Check sheet for the modelled part. Datum: model origin and axes. Units: mm. Coordinates: 2 decimals unless noted, no trailing zeros. Loops run counter-clockwise (first coordinate to the right, second up) from the corner with the lowest first, then second, coordinate; pieces in that order, holes last. Notation, with made-up numbers: (-8.75, 71.25) -> (36.25, 71.25) arc R11 ccw to (36.25, 86.25) -> close; hole circle Ø1 at (52, 67). An arc over 180 degrees is marked (long way). Use one line per item in the form item = value.
from build123d import *

# Parameters (mm, degrees)
F0_W     = 112
F0_H     = 94
F0_W_2   = 3
F0_H_2   = 10
F0_W_3   = 10
F0_H_3   = 3
F0_R     = 1.5
F1_DEPTH = 3


with BuildPart() as f1:
    # F0 (on Front) → F1 (new body)
    with BuildSketch(Plane.XZ):
        Rectangle(F0_W, F0_H)
        with Locations((-51.5, -7)):
            Rectangle(F0_W_2, F0_H_2, mode=Mode.SUBTRACT)
        with Locations((0, -42.5)):
            Rectangle(F0_W_3, F0_H_3, mode=Mode.SUBTRACT)
        with Locations((51.5, -7)):
            Rectangle(F0_W_2, F0_H_2, mode=Mode.SUBTRACT)
        with Locations((-51.5, 3)):
            Circle(F0_R, mode=Mode.SUBTRACT)
        with Locations((-51.5, 13)):
            Rectangle(F0_W_2, F0_H_2, mode=Mode.SUBTRACT)
        with Locations((51.5, 3)):
            Circle(F0_R, mode=Mode.SUBTRACT)
        with Locations((51.5, 13)):
            Rectangle(F0_W_2, F0_H_2, mode=Mode.SUBTRACT)
    extrude(amount=F1_DEPTH)


solid = f1.part
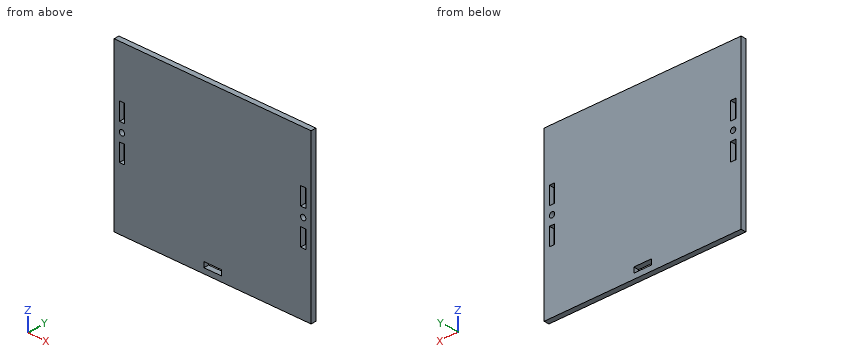
(1) Section check B-B, the plane z = 3. Record the boundary of the cut face in (x, y), plus the area to 3 significant figures.
Established:
outline = (-56, -3) -> (-53, -3) -> (-53, 0) -> (-56, 0) -> close; (-50, -3) -> (50, -3) -> (50, 0) -> (-50, 0) -> close; (53, -3) -> (56, -3) -> (56, 0) -> (53, 0) -> close
area = 318 mm²
(2) Section check D-D, the plane x = -1. Record the boundary of the cut face in (y, z).
Established:
outline = (-3, -47) -> (0, -47) -> (0, -44) -> (-3, -44) -> close; (-3, -41) -> (0, -41) -> (0, 47) -> (-3, 47) -> close
(3) Scan lines: line 1 along Z through (x, y) = (51.5, -2.15); line 2 along X through (y, z) = (-2.45, -7); line 3 along Z through (x, y) = (4, -2.85). Record each from-to range of solid material in increasing order.
Established:
line_1 = -47 to -12, -2 to 1.5, 4.5 to 8, 18 to 47
line_2 = -56 to -53, -50 to 50, 53 to 56
line_3 = -47 to -44, -41 to 47
(4) Section check A-A, the plane x = -51.5. Record the boundary of the cut face in (y, z), plus the area to 3 significant figures.
Established:
outline = (-3, -47) -> (0, -47) -> (0, -12) -> (-3, -12) -> close; (-3, -2) -> (0, -2) -> (0, 1.5) -> (-3, 1.5) -> close; (-3, 4.5) -> (0, 4.5) -> (0, 8) -> (-3, 8) -> close; (-3, 18) -> (0, 18) -> (0, 47) -> (-3, 47) -> close
area = 213 mm²
(5) Section check C-C, the plane y = -1.65. Record the boundary of the cut face in (x, z).
Established:
outline = (-56, -47) -> (56, -47) -> (56, 47) -> (-56, 47) -> close; hole (-53, -12) -> (-50, -12) -> (-50, -2) -> (-53, -2) -> close; hole circle Ø3 at (-51.5, 3); hole (-53, 8) -> (-50, 8) -> (-50, 18) -> (-53, 18) -> close; hole (-5, -44) -> (5, -44) -> (5, -41) -> (-5, -41) -> close; hole (50, -12) -> (53, -12) -> (53, -2) -> (50, -2) -> close; hole circle Ø3 at (51.5, 3); hole (50, 8) -> (53, 8) -> (53, 18) -> (50, 18) -> close
